Read the model definition and answer for the solid it produces. Units are mm, in the model's axes. A direction names the side the tool comes from. Round coordinates to 2 decimals unless told otherwise and drop trailing zeros. Write each loop counter-clockwise with the first axis right and the second up, starting at its lowest first coordinate (ties: lowest second). Pieces come first, ordered by that corner, then holes.
from build123d import *

# Parameters (mm, degrees)
CROQUIS1_W              = 72
CROQUIS1_H              = 40
SALIENTE_EXTRUIR1_DEPTH = 40
CROQUIS5_W              = 16
CROQUIS5_H              = 40
CORTAR_EXTRUIR3_DEPTH   = 32
CROQUIS6_W              = 11.492452947
CROQUIS6_H              = 25
CORTAR_EXTRUIR5_DEPTH   = 16


with BuildPart() as part:
    # Croquis1 → Saliente-Extruir1 (new body)
    with BuildSketch(Plane(origin=(0, 0, 0), x_dir=(1, 0, 0), z_dir=(0, 1, 0))):
        Rectangle(CROQUIS1_W, CROQUIS1_H)
    extrude(amount=SALIENTE_EXTRUIR1_DEPTH)

    # Croquis5 → Cortar-Extruir3 (cut)
    with BuildSketch(Plane(origin=(0, 40, 0), x_dir=(1, 0, 0), z_dir=(0, 1, 0))):
        with Locations((20, 0)):
            Rectangle(CROQUIS5_W, CROQUIS5_H)
    extrude(amount=-CORTAR_EXTRUIR3_DEPTH, mode=Mode.SUBTRACT)

    # Croquis6 → Cortar-Extruir5 (cut)
    with BuildSketch(Plane(origin=(0, 40, 0), x_dir=(1, 0, 0), z_dir=(0, 1, 0))):
        with Locations((-18.746226474, -7.5)):
            Rectangle(CROQUIS6_W, CROQUIS6_H)
    extrude(amount=-CORTAR_EXTRUIR5_DEPTH, mode=Mode.SUBTRACT)


solid = part.part
Q1. Determine the mould class of faces 1 (the flat face through (-1, 20, 20)), 2 (the flat face through (-36, 20, 0)), 3 (the flat face through (-24.492, 32, 8)) for opening direction X: pulls with the +X half, pulls with the -X half, needs draft (parallel to the pull), parting line crosses it, or undercut.
Verdict:
face 1: needs draft
face 2: pulls with the -X half
face 3: undercut
Q2. Section A-A (y = 10) is taken. Determine the outline of the cut face in (x, z).
Verdict:
outline: (-36, -20) - (12, -20) - (12, 20) - (-36, 20) - close; (28, -20) - (36, -20) - (36, 20) - (28, 20) - close
Q3. Which of the six approach directions +Z, -Z, +X, -X, +Y, -Y give full straight-line access (tool end or side, diameter ignored) to faces 4 (the flat face through (36, 20, 0)), 5 (the flat face through (12, 24, 0)), 6 (the flat face through (-19, 32, -5))?
Verdict:
face 4: +Z, -Z, +X, +Y, -Y
face 5: +Z, -Z, +Y
face 6: +Z, +Y
Q4. Flat-ended cylindrical pins translate along their axes: pin 1 Ø8 at (x, y) = (19.5, 33.5) entering from -Z; pin 2 Ø3.5 at (x, y) = (-20.5, 33) entering from +Z. Find the tip coordinate at first contact, or state that the pin passes through.
Verdict:
pin 1: passes through
pin 2: stops at z = -5
Q5. Straight lines are drawn through the part: probe 1 along X at (y, z) = (30.5, 1); probe 2 along X at (y, z) = (23, 18); probe 3 along Y at (x, z) = (-20, -2.5). For each, find the intervals that lie inside material, in ascending order.
Verdict:
probe 1: x = -36 to -24.49, -13 to 12, 28 to 36
probe 2: x = -36 to 12, 28 to 36
probe 3: y = 0 to 24
Q6. Section B-B (z = 8) is taken. Determine the outline of the cut face in (x, y), then the cut area to 3 significant figures.
Verdict:
outline: (-36, 0) - (36, 0) - (36, 40) - (28, 40) - (28, 8) - (12, 8) - (12, 40) - (-13, 40) - (-13, 24) - (-24.49, 24) - (-24.49, 40) - (-36, 40) - close
area: 2,180 mm2
Q7. Section C-C (y = 32.5) is taken. Determine the outline of the cut face in (x, z).
Verdict:
outline: (-36, -20) - (12, -20) - (12, 20) - (-13, 20) - (-13, -5) - (-24.49, -5) - (-24.49, 20) - (-36, 20) - close; (28, -20) - (36, -20) - (36, 20) - (28, 20) - close
Q8. Section D-D (x = -18.5) is taken. Determine the outline of the cut face in (y, z), then the cut area to 3 significant figures.
Verdict:
outline: (0, -20) - (40, -20) - (40, -5) - (24, -5) - (24, 20) - (0, 20) - close
area: 1,200 mm2
